Design review of the part built by this model. Coordinates are the model's own, in mm. A direction names the side the tool comes from. Give positions to 0.01 mm unless a question says otherwise; leave off trailing zeros. Order: outer loops, then holes, each group sorted by start corner. A loop starts at its lowest first (then second) coordinate and runs counter-clockwise, first axis right, second up. Notation, with made-up numbers: (75, 68.25) -> (117, 68.25) arc R37 cw to (117, 106.25) -> close; hole circle Ø8 at (20.5, 73.25). An arc over 180 degrees is marked (long way). One line per item, written item: value. Start each with the question number.
1) For pin 1 (1.6 mm diameter, centred on x = 12, y = 1, fed in from +Z); pin 2 (6 mm diameter, centred on y = 0.5, z = 5.5, fed in from +X); pin 3 (2 mm diameter, centred on x = -16, y = -4, fed in from +Z), all flat-tipped, find the tip position at first contact; note any pin that passes through.
2) Wall thickness on line 1 along Z through (x, y) = (0, 1.5); line 2 along X through (y, z) = (1, -2); line 3 along Z through (x, y) = (-8.5, -2.75): over which ranges is each line inside the solid? List them lowest first. Write a range as from..to.
3) Consider section B-B (x = -5.5). State the section outline as (y, z) points.
4) Consider section C-C (y = 6.25). State the section outline as (x, z) points, plus the area to 3 significant figures.
5) Consider section D-D (y = 2). State the section outline as (x, z) points.
6) Tool access review of faces 5 (the face through (-10, 7.938, -5)), 6 (the face through (12, 0, -1.588)): name each direction out of +Z, -Z, +X, -X, +Y, -Y from which nothing blocks a thin tool from reaching the whole face with its end or side.
7) The part is to be moulded in two halves that separate along Z. For faces 1 (the face through (2.8, 0.111, -12.648)), 2 (the face through (13, 0, 1.588)), 3 (the face through (-10, -7.938, -5)), 4 (the face through (9.845, 0.111, 18.929)), say which applies: released by +Z, released by -Z, zero draft, split by the parting line, or undercut.
8) Consider section A-A (z = 0). State the section outline as (x, y) points.
from build123d import *

# Parameters (mm, degrees)
SKETCH1_R           = 21.336
BOSS_EXTRUDE1_DEPTH = 7.9375


with BuildPart() as part:
    # Sketch1 → Boss-Extrude1 (new body, symmetric)
    with BuildSketch(Plane(origin=(0, 0, 0), x_dir=(1, 0, 0), z_dir=(0, 1, 0))):
        Circle(SKETCH1_R)
        with BuildLine():
            Line((10.806013499, 1.5875), (12.856358728, 1.5875))
            ThreePointArc((12.856358728, 1.5875), (2.578265605, 12.694828178), (-11.218493081, 6.477))
            ThreePointArc((-11.218493081, 6.477), (-12.259404438, 6.198088642), (-12.538315796, 7.239))
            ThreePointArc((-12.538315796, 7.239), (4.50939131, 13.757829553), (14.390702823, -1.5875))
            Line((14.390702823, -1.5875), (10.806013499, -1.5875))
            ThreePointArc((10.806013499, -1.5875), (-10.922, 0), (10.806013499, 1.5875))
        make_face(mode=Mode.SUBTRACT)
    extrude(amount=BOSS_EXTRUDE1_DEPTH, both=True)

    # Sketch2 → Cut-Revolve1 (revolve, cut)
    with BuildSketch(Plane(origin=(0, 0, 0), x_dir=(1, 0, 0), z_dir=(0, 1, 0))):
        Polygon((-0.300030586, 14.474890868), (2.811446909, 13.842963024), (4.246555115, 20.909128764), (1.13507762, 21.541056608), align=None)
    revolve(axis=Axis((2.811446909, 0, -13.842963024), (-0.199032392, 0, 0.979992912)), mode=Mode.SUBTRACT)


solid = part.part
Checked values:
1. pin 1: stops at z = 18.16
1. pin 2: stops at x = 21.19
1. pin 3: stops at z = 15.17
2. line 1: z = -21.34..-14.48, -12.95..-10.92, 10.92..21.34
2. line 2: x = -21.24..-10.74, 10.74..12.8, 14.34..21.24
2. line 3: z = -19.57..-11.72, -9.78..-6.86, 6.86..19.57
3. outline: (-7.94, -20.61) -> (7.94, -20.61) -> (7.94, -13.39) -> (-7.94, -13.39) -> close; (-7.94, -11.73) -> (7.94, -11.73) -> (7.94, -9.44) -> (-7.94, -9.44) -> close; (-7.94, 9.44) -> (7.94, 9.44) -> (7.94, 20.61) -> (-7.94, 20.61) -> close
4. outline: circle Ø42.67 at (0, 0); hole (-12.54, -7.24) arc R14.48 ccw to (14.39, 1.59) -> (10.81, 1.59) arc R10.92 ccw (long way) to (10.81, -1.59) -> (12.86, -1.59) arc R12.95 cw to (-11.22, -6.48) arc R0.76 ccw to start
4. area: 991 mm^2
5. outline: (-12.54, -7.24) arc R0.76 cw to (-11.22, -6.48) arc R12.95 ccw to (12.86, -1.59) -> (10.81, -1.59) arc R10.92 cw (long way) to (10.81, 1.59) -> (14.39, 1.59) arc R14.48 cw to (5.26, -13.49) -> (6.63, -20.28) arc R21.34 ccw (long way) to (1.8, -21.26) -> (0.42, -14.47) arc R14.48 cw to start
6. face 5: +Z, -Z, +X, -X, +Y
6. face 6: +Y, -Y
7. face 1: undercut
7. face 2: undercut
7. face 3: zero draft
7. face 4: split by the parting line
8. outline: (-21.34, -7.94) -> (-10.92, -7.94) -> (-10.92, 7.94) -> (-21.34, 7.94) -> close; (14.48, -7.94) -> (21.34, -7.94) -> (21.34, 7.94) -> (14.48, 7.94) -> close
